Check sheet for the drawn part. Datum: minimum x, y, z corner. Units: mm. A direction names the side the tool comes from. Give positions to 0.01 mm unless a question says otherwise; leave off trailing zeros. Write each loop counter-clockwise with the first axis right and the second up, starting at its lowest first coordinate (ties: lowest second). Pieces come first, ordered by that corner, then holes. Notation, with made-up numbers: M 44,-30.75 L 70,-30.75 A25 cw 70,-15.75 Z; hole C -4,33.25 d6. An arc over 180 degrees is marked long. Write item = value, one per line. Start each with the question number.
1) Gauge pin test, flat ends, axial feed: pin 1 (5 mm diameter, centred on x = 18.5, y = 19.5, fed in from +Z); pin 2 (1.5 mm diameter, centred on x = 6.5, z = 7, fed in from -Y); pin 3 (5 mm diameter, centred on x = 11, y = 11, fed in from -Z); pin 4 (5 mm diameter, centred on x = 16, z = 9.5, fed in from -Y). Record the tip position at first contact, or that the pin passes through.
2) Sectioned sample at C-C, the plane y = 8.25. Record the cut outline in (x, z), then the cut area to 3 significant figures.
3) Draft check along Y on the marked faces 1, 2, 3 and 4. Enter one of: pulls with the +Y half, pulls with the -Y half, needs draft (parallel to the pull), parting line crosses it, or undercut.
4) Sectioned sample at D-D, the plane x = 2.75. Record the cut outline in (y, z).
5) Set-up check for the marked faces 5 and 6: record each of +Z, -Z, +X, -X, +Y, -Y from which the full face is reachable in a straight line by a thin tool's end or side.
6) Sectioned sample at A-A, the plane x = 11. Record the cut outline in (y, z).
7) Scan lines: L1, parallel to Y at x = 11, z = 1; L2, parallel to X at y = 11, z = 6.25; L3, parallel to Z at x = 4.5, y = 16.25. Record each from-to range of solid material in increasing order.
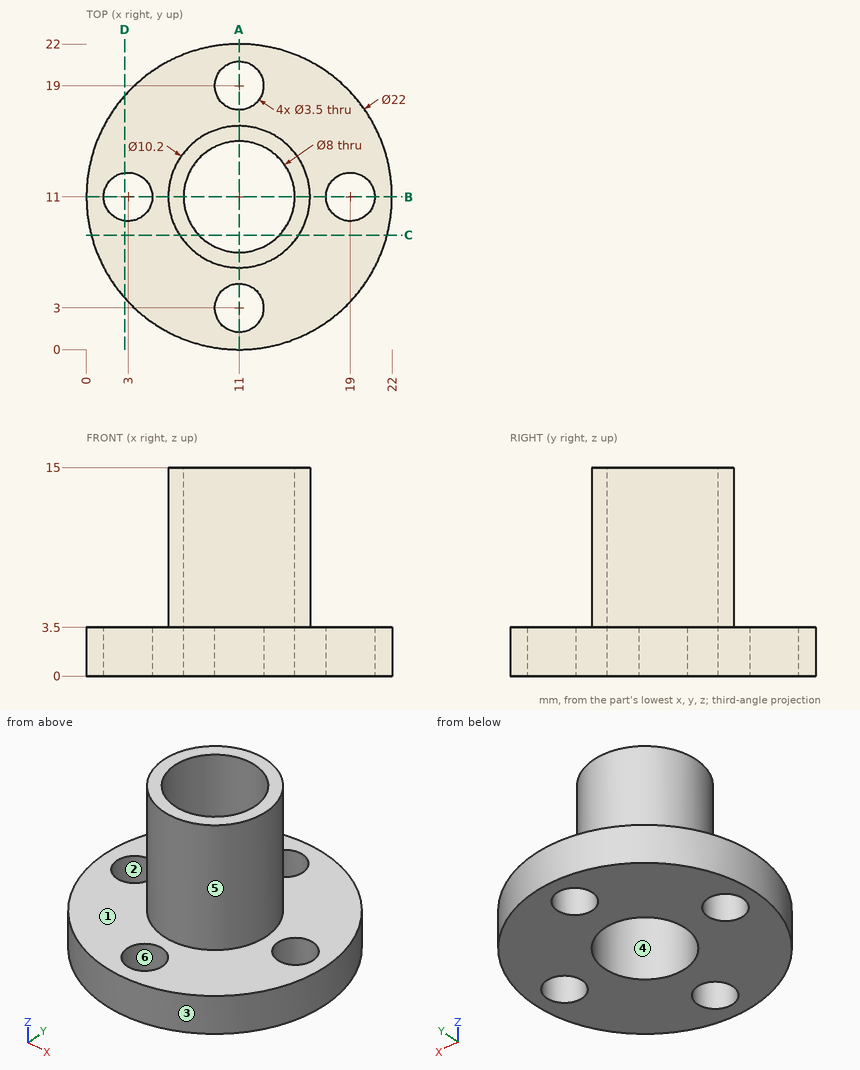
Data:
q1.pin_1 = 3.5
q1.pin_2 = 7.54
q1.pin_3 = through
q1.pin_4 = 6.55
q2.outline = M 0.35,0 L 8.1,0 L 8.1,15 L 6.7,15 L 6.7,3.5 L 0.35,3.5 Z; M 13.9,0 L 21.65,0 L 21.65,3.5 L 15.3,3.5 L 15.3,15 L 13.9,15 Z
q2.area = 86.2 mm2
q3.face_1 = needs draft
q3.face_2 = undercut
q3.face_3 = parting line crosses it
q3.face_4 = undercut
q4.outline = M 3.72,0 L 9.27,0 L 9.27,3.5 L 3.72,3.5 Z; M 12.73,0 L 18.28,0 L 18.28,3.5 L 12.73,3.5 Z
q5.face_5 = +Z
q5.face_6 = +Z, -Z
q6.outline = M 0,0 L 1.25,0 L 1.25,3.5 L 0,3.5 Z; M 4.75,0 L 7,0 L 7,15 L 5.9,15 L 5.9,3.5 L 4.75,3.5 Z; M 15,0 L 17.25,0 L 17.25,3.5 L 16.1,3.5 L 16.1,15 L 15,15 Z; M 20.75,0 L 22,0 L 22,3.5 L 20.75,3.5 Z
q7.L1 = 0 to 1.25, 4.75 to 7, 15 to 17.25, 20.75 to 22
q7.L2 = 5.9 to 7, 15 to 16.1
q7.L3 = 0 to 3.5
